The listing builds one solid part. Answer for the finished solid, in the listing's coordinates (mm). Face numbers are marked on the shaded views. A direction names the side the tool comes from. Round coordinates to 2 decimals unless told otherwise and drop trailing zeros. Order: outer loops, then holes, each group sorted by start corner. A loop starts at its lowest first (then second) coordinate and runs counter-clockwise, first axis right, second up. Notation, with made-up numbers: (6, -17.5) - (17, -17.5) arc R9 ccw to (17, -2.5) - close; hole circle Ø9 at (-25, 49). An arc over 180 degrees is marked (long way). Use CSV: the item, a comma, the result in double quotes. Start each with the question number.
Item 1: Determine the mould class of the marked faces 1, 2 and 3 for opening direction X: +X half, -X half, draft (parallel to the pull), parting line (faces both ways), or undercut.
Item 2: Find section A-A, the plane x = -417. Give the vertices of the cut face in (y, z).
Item 3: Flat-ended cylindrical pins translate along their axes: P1, Ø2, axis at x = -604, y = 7.5, coming from the +Z side; P2, Ø6, axis at x = -468.5, y = 58.5, coming from the -Z side; P3, Ø1.5, axis at x = -547, y = 107.5, coming from the +Z side. Find the tip coordinate at first contact, or state that the pin passes through.
Item 4: Find section B-B, the plane y = 50.5. Give the vertices of the cut face in (x, z).
Item 5: Find section C-C, the plane x = -97. Give the vertices of the cut face in (y, z).
Item 6: Find section D-D, the plane z = 163. Give the vertices of the cut face in (x, y).
Item 7: For the marked faces 4, 5 and 6, determine the directions among +Z, -Z, +X, -X, +Y, -Y from which every point of the face is accessible in a straight line to the end or side of a thin tool.
Item 8: Straight lines are drawn through the part: line 1 along X through (y, z) = (76, 737); line 2 along Y through (x, z) = (-481.5, 507); line 3 along X through (y, z) = (138, 618). For each, find the intervals that lie inside material, in ascending order. Write a range as [from, to].
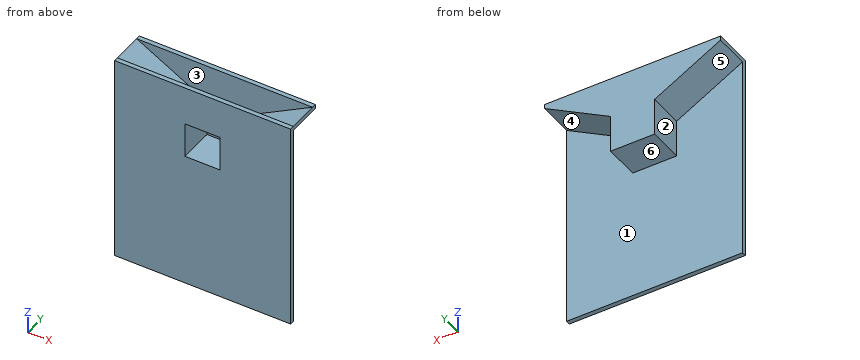
```python
from build123d import *

# Parameters (mm, degrees)
F1_DEPTH = 19.05
F2_DEPTH = 152.4
F4_DEPTH = 19.05


with BuildPart() as f1:
    # F0 (on Front) → F1 (new body)
    with BuildSketch(Plane.XZ):
        Polygon((-762, 0), (0, 0), (0, 895.35), (-285.75, 737.693186), (-285.75, 593.832731), (-285.75, 574.782731), (-476.25, 574.782731), (-476.25, 593.832731), (-476.25, 737.693186), (-762, 895.35), align=None)
        Polygon((-304.8, 746.232731), (0, 914.4), (-762, 914.4), (-457.2, 746.232731), align=None)
        Polygon((-285.75, 737.693186), (0, 895.35), (0, 914.4), (-304.8, 746.232731), (-304.8, 593.832731), (-457.2, 593.832731), (-457.2, 746.232731), (-762, 914.4), (-762, 895.35), (-476.25, 737.693186), (-476.25, 593.832731), (-476.25, 574.782731), (-285.75, 574.782731), (-285.75, 593.832731), align=None)
    extrude(amount=F1_DEPTH)

    # F0 (on Front) → F2 (join)
    with BuildSketch(Plane.XZ):
        Polygon((-285.75, 737.693186), (0, 895.35), (0, 914.4), (-304.8, 746.232731), (-304.8, 593.832731), (-457.2, 593.832731), (-457.2, 746.232731), (-762, 914.4), (-762, 895.35), (-476.25, 737.693186), (-476.25, 593.832731), (-476.25, 574.782731), (-285.75, 574.782731), (-285.75, 593.832731), align=None)
    extrude(amount=-F2_DEPTH)

    # F3 (on face) → F4 (join)
    with BuildSketch(Plane(origin=(0, 152.4, 0), x_dir=(-1, 0, 0), z_dir=(0, 1, 0))):
        Polygon((762, 914.4), (0, 914.4), (304.8, 746.232731), (304.8, 593.832731), (457.2, 593.832731), (457.2, 746.232731), align=None)
    extrude(amount=-F4_DEPTH)


solid = f1.part
```
Worked out:
1,face 1,"draft"
1,face 2,"-X half"
1,face 3,"undercut"
2,outline,"(-19.05, 0) - (0, 0) - (0, 574.78) - (152.4, 574.78) - (152.4, 914.4) - (133.35, 914.4) - (133.35, 593.83) - (-19.05, 593.83) - close; (-19.05, 746.23) - (0, 746.23) - (0, 914.4) - (-19.05, 914.4) - close"
3,P1,"stops at z = 827.78"
3,P2,"stops at z = 574.78"
3,P3,"stops at z = 796.19"
4,outline,"(-762, 895.35) - (-476.25, 737.69) - (-476.25, 574.78) - (-285.75, 574.78) - (-285.75, 737.69) - (0, 895.35) - (0, 914.4) - (-304.8, 746.23) - (-304.8, 593.83) - (-457.2, 593.83) - (-457.2, 746.23) - (-762, 914.4) - close"
5,outline,"(-19.05, 0) - (0, 0) - (0, 841.83) - (152.4, 841.83) - (152.4, 914.4) - (133.35, 914.4) - (133.35, 860.88) - (0, 860.88) - (0, 914.4) - (-19.05, 914.4) - close"
6,outline,"(-762, -19.05) - (0, -19.05) - (0, 0) - (-762, 0) - close"
7,face 4,"-Z, +X, +Y"
7,face 5,"-Z, -X, +Y"
7,face 6,"-Z, +X, -X, +Y"
8,line 1,"x = [-476.25, -457.2], [-304.8, -285.75]"
8,line 2,"y = [-19.05, 0]"
8,line 3,"x = [-476.25, -285.75]"
